from build123d import *

# Parameters (mm, degrees)
F1_DEPTH       = 12
F3_DEPTH       = 4
F5_D           = 2.2
F5_DEPTH       = 10
F5_CSINK_D     = 2.5
F5_CSINK_ANGLE = 90
F5_TIP         = 0.6609466809
F6_D           = 2.2
F6_DEPTH       = 10
F6_CSINK_D     = 2.5
F6_CSINK_ANGLE = 90
F6_TIP         = 0.6609466809
F7_D           = 2.2
F7_DEPTH       = 10
F7_CSINK_D     = 2.5
F7_CSINK_ANGLE = 90
F7_TIP         = 0.6609466809
F8_D           = 2.2
F8_DEPTH       = 10
F8_CSINK_D     = 2.5
F8_CSINK_ANGLE = 90
F8_TIP         = 0.6609466809


with BuildPart() as f1:
    # F0 (on Top) → F1 (new body)
    with BuildSketch(Plane.XY):
        with BuildLine():
            Line((41.2117568254, 36.543219165), (-33.2882431746, 36.543219165))
            ThreePointArc((-33.2882431746, 36.543219165), (-35.0560101275, 35.810986118), (-35.7882431746, 34.043219165))
            Line((-35.7882431746, 34.043219165), (-35.7882431746, -40.456780835))
            ThreePointArc((-35.7882431746, -40.456780835), (-35.0560101275, -42.2245477879), (-33.2882431746, -42.956780835))
            Line((-33.2882431746, -42.956780835), (-18.7882431746, -42.956780835))
            ThreePointArc((-18.7882431746, -42.956780835), (-17.0204762216, -42.2245477879), (-16.2882431746, -40.456780835))
            Line((-16.2882431746, -40.456780835), (-16.2882431746, 14.543219165))
            ThreePointArc((-16.2882431746, 14.543219165), (-15.5560101275, 16.310986118), (-13.7882431746, 17.043219165))
            Line((-13.7882431746, 17.043219165), (41.2117568254, 17.043219165))
            ThreePointArc((41.2117568254, 17.043219165), (42.9795237784, 17.7754522121), (43.7117568254, 19.543219165))
            Line((43.7117568254, 19.543219165), (43.7117568254, 34.043219165))
            ThreePointArc((43.7117568254, 34.043219165), (42.9795237784, 35.810986118), (41.2117568254, 36.543219165))
        make_face()
    extrude(amount=F1_DEPTH)

    # F2 (on face) → F3 (join)
    with BuildSketch(Plane.XY.offset(12)):
        with BuildLine():
            ThreePointArc((-33.9882431746, 33.243219165), (-33.5489033463, 34.3038793368), (-32.4882431746, 34.743219165))
            Line((-32.4882431746, 34.743219165), (41.2117568254, 34.743219165))
            Line((41.2117568254, 34.743219165), (41.2117568254, 36.543219165))
            Line((41.2117568254, 36.543219165), (-33.2882431746, 36.543219165))
            ThreePointArc((-33.2882431746, 36.543219165), (-35.0560101275, 35.810986118), (-35.7882431746, 34.043219165))
            Line((-35.7882431746, 34.043219165), (-35.7882431746, -40.456780835))
            Line((-35.7882431746, -40.456780835), (-33.9882431746, -40.456780835))
            Line((-33.9882431746, -40.456780835), (-33.9882431746, 33.243219165))
        make_face()
    extrude(amount=F3_DEPTH)

    # F5
    with Locations(Plane(origin=(0, 0, 0), x_dir=(1, 0, 0), z_dir=(0, 0, -1))):
        with Locations((34.7117568254, -26.043219165)):
            CounterSinkHole(F5_D / 2, F5_CSINK_D / 2, depth=F5_DEPTH, counter_sink_angle=F5_CSINK_ANGLE)
            with Locations((0, 0, -(F5_DEPTH + F5_TIP / 2))):  # 118° drill point
                Cone(0, F5_D / 2, F5_TIP, mode=Mode.SUBTRACT)

    # F6
    with Locations(Plane(origin=(0, 0, 0), x_dir=(1, 0, 0), z_dir=(0, 0, -1))):
        with Locations((-15.2882431746, -26.043219165)):
            CounterSinkHole(F6_D / 2, F6_CSINK_D / 2, depth=F6_DEPTH, counter_sink_angle=F6_CSINK_ANGLE)
            with Locations((0, 0, -(F6_DEPTH + F6_TIP / 2))):  # 118° drill point
                Cone(0, F6_D / 2, F6_TIP, mode=Mode.SUBTRACT)

    # F7
    with Locations(Plane(origin=(0, 0, 0), x_dir=(1, 0, 0), z_dir=(0, 0, -1))):
        with Locations((-25.2882431746, -16.043219165)):
            CounterSinkHole(F7_D / 2, F7_CSINK_D / 2, depth=F7_DEPTH, counter_sink_angle=F7_CSINK_ANGLE)
            with Locations((0, 0, -(F7_DEPTH + F7_TIP / 2))):  # 118° drill point
                Cone(0, F7_D / 2, F7_TIP, mode=Mode.SUBTRACT)

    # F8
    with Locations(Plane(origin=(0, 0, 0), x_dir=(1, 0, 0), z_dir=(0, 0, -1))):
        with Locations((-25.2882431746, 33.956780835)):
            CounterSinkHole(F8_D / 2, F8_CSINK_D / 2, depth=F8_DEPTH, counter_sink_angle=F8_CSINK_ANGLE)
            with Locations((0, 0, -(F8_DEPTH + F8_TIP / 2))):  # 118° drill point
                Cone(0, F8_D / 2, F8_TIP, mode=Mode.SUBTRACT)


solid = f1.part
Can you work these out from the model? Positions are in its coordinate system, mm. A direction names the side the tool comes from. Coordinates: 2 decimals unless noted, no trailing zeros. Write each loop counter-clockwise with the first axis right and the second up, starting at its lowest first coordinate (ties: lowest second). Pieces come first, ordered by that corner, then holes.
Q1. Imagine slicing it at D-D, the plane z = 6.75. List the corners of the cut face in (x, y) for me, plus the area to 3 significant figures.
Results found:
outline: (-35.79, -40.46) arc R2.5 ccw to (-33.29, -42.96) - (-18.79, -42.96) arc R2.5 ccw to (-16.29, -40.46) - (-16.29, 14.54) arc R2.5 cw to (-13.79, 17.04) - (41.21, 17.04) arc R2.5 ccw to (43.71, 19.54) - (43.71, 34.04) arc R2.5 ccw to (41.21, 36.54) - (-33.29, 36.54) arc R2.5 ccw to (-35.79, 34.04) - close; hole circle Ø2.2 at (-25.29, -33.96); hole circle Ø2.2 at (-25.29, 16.04); hole circle Ø2.2 at (-15.29, 26.04); hole circle Ø2.2 at (34.71, 26.04)
area: 2,700 mm2
Q2. Please list where these lines run through material, in increasing order: L1, parallel to Z at x = -10, y = 24; L2, parallel to X at y = -30, z = 1.5; L3, parallel to X at y = 27, z = 15.5.
Results found:
L1: z = 0 to 12
L2: x = -35.79 to -16.29
L3: x = -35.79 to -33.99
Q3. Imagine slicing it at A-A, the plane y = 30. List the corners of the cut face in (x, z) for me.
Results found:
outline: (-35.79, 0) - (43.71, 0) - (43.71, 12) - (-33.99, 12) - (-33.99, 16) - (-35.79, 16) - close
Q4. If we mould it in two halves opening along Y, with no side actions, what happens to faces 4 (the face through (13, 17.043, 6)), 5 (the face through (-25.2, -33.787, 10.546)), 6 (the face through (41.212, 36, 14))? For each: +Y half, -Y half, draft (parallel to the pull), parting line (faces both ways), or undercut.
Results found:
face 4: -Y half
face 5: undercut
face 6: draft
Q5. Imagine slicing it at B-B, the plane z = 14.5. List the corners of the cut face in (x, y) for me, plus the area to 3 significant figures.
Results found:
outline: (-35.79, -40.46) - (-33.99, -40.46) - (-33.99, 33.24) arc R1.5 cw to (-32.49, 34.74) - (41.21, 34.74) - (41.21, 36.54) - (-33.29, 36.54) arc R2.5 ccw to (-35.79, 34.04) - close
area: 273 mm2
Q6. Imagine slicing it at C-C, the plane x = -9.5. List the corners of the cut face in (y, z) for me.
Results found:
outline: (17.04, 0) - (36.54, 0) - (36.54, 16) - (34.74, 16) - (34.74, 12) - (17.04, 12) - close
Q7. For P1, Ø3, axis at x = 1, z = 14, coming from the -Y side; P2, Ø2, axis at y = -11, z = 13.5, coming from the +X side; P3, Ø0.5, axis at y = 36, z = 13, coming from the +X side, each with a flat end and sliding along its axis, tell me the tip position at first contact or that it passes through.
Results found:
P1: stops at y = 34.74
P2: stops at x = -33.99
P3: stops at x = 41.21
Q8. Which directions (+Z, -Z, +X, -X, +Y, -Y) give clear straight access to the entire face, cutting with the end or side of a thin tool? Please do faces 1 (the face through (-35, -40.457, 14)), 2 (the face through (-15.575, 16.291, 5.916)), 3 (the face through (-24.415, 16.713, 5.144)).
Results found:
face 1: +Z, +X, -X, -Y
face 2: +Z, -Z, +X, -Y
face 3: -Z
